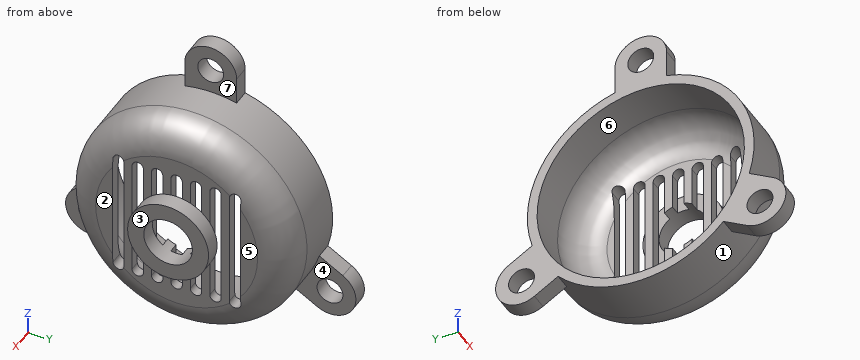
```python
from build123d import *

# Parameters (mm, degrees)
BOSS_EXTRUDE1_START = 5
SKETCH3_R           = 4
BOSS_EXTRUDE1_DEPTH = 5
CIRPATTERN1_COUNT   = 3
CUT_EXTRUDE1_DEPTH  = 5


with BuildPart() as part:
    # Sketch2 → Revolve1 (revolve)
    with BuildSketch(Plane(origin=(0, 0, 0), x_dir=(-1, 0, 0), z_dir=(0, 1, 0)), mode=Mode.PRIVATE) as revolve1_sk:
        with BuildLine():
            Line((-12, 32), (0, 32))
            Line((0, 32), (0, 35))
            Line((0, 35), (-15, 35))
            ThreePointArc((-15, 35), (-22.071067812, 32.071067812), (-25, 25))
            Line((-25, 25), (-25, 12.5))
            Line((-25, 12.5), (-22, 12.5))
            Line((-22, 12.5), (-22, 22))
            ThreePointArc((-22, 22), (-19.071067812, 29.071067812), (-12, 32))
        make_face()
        Polygon((-22, 7.5), (-22, 12.5), (-25, 12.5), (-30, 12.5), (-30, 7.5), align=None)
    revolve(revolve1_sk.sketch.rotate(Axis((0, 0, 0), (-1, 0, 0)), 180), axis=Axis((0, 0, 0), (-1, 0, 0)))

    # Sketch3 → Boss-Extrude1 (add)
    with BuildSketch(Plane.YZ.offset(BOSS_EXTRUDE1_START)):
        with BuildLine():
            Line((8, 34.073450075), (8, 42.5))
            ThreePointArc((8, 42.5), (0, 50.5), (-8, 42.5))
            Line((-8, 42.5), (-8, 34.073450075))
            ThreePointArc((-8, 34.073450075), (0, 35), (8, 34.073450075))
        make_face()
        with Locations(Location((0, 42.5, 0), (0, 0, 270))):
            Circle(SKETCH3_R, mode=Mode.SUBTRACT)
    boss_extrude1 = extrude(amount=-BOSS_EXTRUDE1_DEPTH)

    # CirPattern1: Boss-Extrude1 ×3 about axis
    cirpattern1_axis = Axis((0, 0, 0), (1, 0, 0))
    for i in range(1, CIRPATTERN1_COUNT):
        add(boss_extrude1.rotate(cirpattern1_axis, i * 360 / CIRPATTERN1_COUNT))

    # Sketch4 → Cut-Extrude1 (cut)
    with BuildSketch(Plane.YZ.offset(25)):
        with BuildLine():
            Line((1.75, 18.25), (1.75, -18.25))
            ThreePointArc((1.75, -18.25), (0, -20), (-1.75, -18.25))
            Line((-1.75, -18.25), (-1.75, 18.25))
            ThreePointArc((-1.75, 18.25), (0, 20), (1.75, 18.25))
        make_face()
        with BuildLine():
            Line((7.75, 18.25), (7.75, -18.25))
            ThreePointArc((7.75, -18.25), (6, -20), (4.25, -18.25))
            Line((4.25, -18.25), (4.25, 18.25))
            ThreePointArc((4.25, 18.25), (6, 20), (7.75, 18.25))
        make_face()
        with BuildLine():
            Line((13.75, 18.25), (13.75, -18.25))
            ThreePointArc((13.75, -18.25), (12, -20), (10.25, -18.25))
            Line((10.25, -18.25), (10.25, 18.25))
            ThreePointArc((10.25, 18.25), (12, 20), (13.75, 18.25))
        make_face()
        with BuildLine():
            Line((19.75, 18.25), (19.75, -18.25))
            ThreePointArc((19.75, -18.25), (18, -20), (16.25, -18.25))
            Line((16.25, -18.25), (16.25, 18.25))
            ThreePointArc((16.25, 18.25), (18, 20), (19.75, 18.25))
        make_face()
        with BuildLine():
            Line((-4.25, 18.25), (-4.25, -18.25))
            ThreePointArc((-4.25, -18.25), (-6, -20), (-7.75, -18.25))
            Line((-7.75, -18.25), (-7.75, 18.25))
            ThreePointArc((-7.75, 18.25), (-6, 20), (-4.25, 18.25))
        make_face()
        with BuildLine():
            Line((-10.25, 18.25), (-10.25, -18.25))
            ThreePointArc((-10.25, -18.25), (-12, -20), (-13.75, -18.25))
            Line((-13.75, -18.25), (-13.75, 18.25))
            ThreePointArc((-13.75, 18.25), (-12, 20), (-10.25, 18.25))
        make_face()
        with BuildLine():
            Line((-16.25, 18.25), (-16.25, -18.25))
            ThreePointArc((-16.25, -18.25), (-18, -20), (-19.75, -18.25))
            Line((-19.75, -18.25), (-19.75, 18.25))
            ThreePointArc((-19.75, 18.25), (-18, 20), (-16.25, 18.25))
        make_face()
    extrude(amount=-CUT_EXTRUDE1_DEPTH, mode=Mode.SUBTRACT)


solid = part.part
```
The model under review builds one solid part; all positions refer to its coordinate system, in mm. Face numbers are marked on the shaded views. A direction names the side the tool comes from. Round coordinates to 2 decimals unless told otherwise and drop trailing zeros. Order: outer loops, then holes, each group sorted by start corner. A loop starts at its lowest first (then second) coordinate and runs counter-clockwise, first axis right, second up. Notation, with made-up numbers: (19, -6.5) -> (60, -6.5) arc R23 ccw to (60, 16.5) -> close; hole circle Ø4 at (-9.5, -34.5). An arc over 180 degrees is marked (long way). One line per item, written item: value. Start each with the question number.
Q1. Take a section at A-A (y = 38). Write out the cut boundary in (x, z).
Q2. Machinability: for the marked faces 1, 2, 3, 4 and 5, which of the approach directions +Z, -Z, +X, -X, +Y, -Y give a long, thin tool a straight path to every point of the face, cutting with its end or side? Answer none if there is none.
Q3. Wall thickness on line 1 (Y direction, x = 26.75, z = 0); line 2 (Z direction, x = 2, y = -37.5); line 3 (X direction, y = 41.5, z = -16.5): over which ranges is each line inside the solid? List them lowest first.
Q4. Mouldability with a two-part tool opening along Y and no side actions: class the marked faces 6 and 7 as released by +Y, released by -Y, zero draft, split by the parting line, or undercut.
Q5. Take a section at B-B (z = 0). Count the separate pieces of the cut face and the enclosed holes in it, and give its area (4 significant figures).
Q6. Clearance check with flat-ended pins moving along their axes: pin 1 Ø1.1 at (y, z) = (-20.5, 3.5) entering from -X; pin 2 Ø1.6 at (y, z) = (23, 6) entering from +X; pin 3 Ø3 at (x, y) = (25, 8) entering from +Z; pin 4 Ø7 at (y, z) = (0, 42.5) entering from +X. State where each tip first meets the part, or that it passes through.
Reported:
1. outline: (0, -29.16) -> (5, -29.16) -> (5, -25.07) -> (0, -25.07) -> close; (0, -17.43) -> (5, -17.43) -> (5, -12.7) -> (0, -12.7) -> close
2. face 1: +X
2. face 2: +Z, -Z, +X, -Y
2. face 3: +Z, -Z, +X, +Y, -Y
2. face 4: -Z, +X, +Y
2. face 5: +Z, -Z, +X, +Y
3. line 1: y = -12.5 to -7.5, 7.5 to 12.5
3. line 2: z = -29.22 to -25.19, -17.31 to -12.41
3. line 3: x = 0 to 5
4. face 6: undercut
4. face 7: zero draft
5. separate pieces: 6
5. enclosed holes: 0
5. area: 303.5 mm2
6. pin 1: stops at x = 22
6. pin 2: stops at x = 25
6. pin 3: stops at z = 29.22
6. pin 4: passes through
